CAD build for the part. Positions are in the model's coordinates, mm. A direction names the side the tool comes from. Round coordinates to 2 decimals unless told otherwise and drop trailing zeros. Write each loop counter-clockwise with the first axis right and the second up, starting at its lowest first coordinate (ties: lowest second). Pieces come first, ordered by that corner, then holes. Notation, with made-up numbers: (58, 68.5) - (99, 68.5) arc R15 ccw to (99, 93.5) - close; hole circle Ø4 at (-11, 27). An arc over 180 degrees is marked (long way). Put each result on its own line as item: value. Start each with the question number.
Item 1: Pin check, flat tips, straight feed: pin 1 Ø8 at (x, y) = (-13, 6) entering from -Z; pin 2 Ø6 at (y, z) = (8, 6.5) entering from -X; pin 3 Ø1.5 at (x, z) = (12.5, 10.5) entering from -Y; pin 4 Ø10.5 at (x, z) = (-2.5, 4) entering from +Y. Stop position of each tip, or through.
Item 2: Cut at C-C (y = 7.75). Give the cut face in (x, z), and give its area (3 significant figures).
Item 3: 3-axis set-ups, long thin cutter, end or side, ignore diameter. For faces 1 (the flat face through (0, 0, 0)), 2 (the flat face through (0, 2, 0)): which of +Z, -Z, +X, -X, +Y, -Y reach the whole face in a straight line?
Item 4: Mould opens along X. For faces 3 (the flat face through (-11, 15, 8)), 4 (the cylindrical face through (-10.648, 7.395, -13.887)), 5 (the cylindrical face through (3.755, 9.423, 11.923)) say: released by +X, released by -X, zero draft, split by the parting line, or undercut.
Item 5: Cut at D-D (y = 2.75). Give the cut face in (x, z), and give its area (3 significant figures).
Item 6: Drill centre lines: line 1 (X direction, y = 11.75, z = 0); line 2 (Y direction, x = -4, z = 7); line 3 (Z direction, x = -2, y = 3.5). Where is each one in solid material? Low to high. Write a range as from..to.
Item 7: Cut at B-B (x = 0). Give the cut face in (y, z).
Item 8: Cut at A-A (z = 0). Give the cut face in (x, y), and give its area (3 significant figures).
```python
from build123d import *

# Parameters (mm, degrees)
SKETCH1_R           = 17.5
SKETCH1_R_2         = 12.5
BOSS_EXTRUDE1_DEPTH = 15
SKETCH2_R           = 12.5
BOSS_EXTRUDE2_DEPTH = 2
FILLET1_R           = 2


with BuildPart() as part:
    # Sketch1 → Boss-Extrude1 (new body)
    with BuildSketch(Plane(origin=(0, 0, 0), x_dir=(1, 0, 0), z_dir=(0, 1, 0))):
        with Locations(Location((0, 0, 0), (0, 0, 270))):
            Circle(SKETCH1_R)
        with Locations(Location((0, 0, 0), (0, 0, 270))):
            Circle(SKETCH1_R_2, mode=Mode.SUBTRACT)
    extrude(amount=BOSS_EXTRUDE1_DEPTH)

    # Sketch2 → Boss-Extrude2 (add)
    with BuildSketch(Plane.XZ):
        with Locations(Location((0, 0, 0), (0, 0, 270))):
            Circle(SKETCH2_R)
    extrude(amount=-BOSS_EXTRUDE2_DEPTH)

    # Fillet1
    fillet1_edges = [part.edges().sort_by_distance(p)[0] for p in [
        (0, 2, -12.5),
    ]]
    fillet(fillet1_edges, radius=FILLET1_R)


solid = part.part
```
Output values:
1. pin 1: z = -15.01
1. pin 2: x = -17.15
1. pin 3: y = 0
1. pin 4: y = 2
2. outline: circle Ø35 at (0, 0); hole circle Ø25 at (0, 0)
2. area: 471 mm2
3. face 1: +Z, -Z, +X, -X, -Y
3. face 2: +Y
4. face 3: zero draft
4. face 4: split by the parting line
4. face 5: undercut
5. outline: circle Ø35 at (0, 0); hole circle Ø24.12 at (0, 0)
5. area: 505 mm2
6. line 1: -17.5..-12.5, 12.5..17.5
6. line 2: 0..2
6. line 3: -17.39..-12.27, 12.27..17.39
7. outline: (0, -17.5) - (15, -17.5) - (15, -12.5) - (4, -12.5) arc R2 cw to (2, -10.5) - (2, 10.5) arc R2 cw to (4, 12.5) - (15, 12.5) - (15, 17.5) - (0, 17.5) - close
8. outline: (-17.5, 0) - (17.5, 0) - (17.5, 15) - (12.5, 15) - (12.5, 4) arc R2 cw to (10.5, 2) - (-10.5, 2) arc R2 cw to (-12.5, 4) - (-12.5, 15) - (-17.5, 15) - close
8. area: 202 mm2
